Here's how the part is built. I have some questions about the finished solid (model axes, mm). A direction names the side the tool comes from. Round coordinates to 2 decimals unless told otherwise and drop trailing zeros. Write each loop counter-clockwise with the first axis right and the second up, starting at its lowest first coordinate (ties: lowest second). Pieces come first, ordered by that corner, then holes. Notation, with made-up numbers: (45.5, 40.25) -> (77.5, 40.25) arc R8 cw to (77.5, 45.25) -> close; hole circle Ø2 at (-11, 47). An arc over 180 degrees is marked (long way). Answer in a Markdown table with one row per item. Add a question column.
from build123d import *

# Parameters (mm, degrees)
SKETCH1_R           = 3.25
BOSS_EXTRUDE1_DEPTH = 10
SKETCH2_R           = 1.75
CUT_EXTRUDE1_DEPTH  = 2.5
SKETCH6_R           = 5
BOSS_EXTRUDE2_DEPTH = 5
BOSS_EXTRUDE3_DEPTH = 1


with BuildPart() as part:
    # Sketch1 → Boss-Extrude1 (new body)
    with BuildSketch(Plane(origin=(0, 0, 0), x_dir=(1, 0, 0), z_dir=(0, 1, 0))):
        Circle(SKETCH1_R)
    extrude(amount=BOSS_EXTRUDE1_DEPTH)

    # Sketch2 → Cut-Extrude1 (cut)
    with BuildSketch(Plane.XZ):
        Circle(SKETCH2_R)
    extrude(amount=-CUT_EXTRUDE1_DEPTH, mode=Mode.SUBTRACT)

    # Sketch6 → Boss-Extrude2 (add)
    with BuildSketch(Plane(origin=(0, 10, 0), x_dir=(1, 0, 0), z_dir=(0, 1, 0))):
        Circle(SKETCH6_R)
    extrude(amount=BOSS_EXTRUDE2_DEPTH)

    # Sketch9 → Boss-Extrude3 (add)
    with BuildSketch(Plane(origin=(0, 15, 0), x_dir=(1, 0, 0), z_dir=(0, 1, 0))):
        Polygon((-2.9, 2.9), (-2.9, -2.9), (2.9, 0), align=None)
    extrude(amount=BOSS_EXTRUDE3_DEPTH)


solid = part.part
Item 1: If we section it at C-C on y = 3.75: Please give me the cut outline in (x, z), then the cut area to 3 significant figures.
Item 2: On a 3-axis mill with a long thin cutter (end or side, diameter ignored), from which of +Z, -Z, +X, -X, +Y, -Y can I reach the whole of each face in a straight line? I mean faces 1 (the flat face through (1.4, 0, 1.4)), 2 (the flat face through (-2.9, 15.5, 0)), 3 (the flat face through (-1, 16, 0)), 4 (the flat face through (1, 10, 3.3)), 5 (the flat face through (0.04, 15.49, -1.43)). Say none if no direction works.
Item 3: If we section it at A-A on x = 0: Please give me the cut outline in (y, z).
Item 4: I need wall thicknesses on line 1 along Z through (x, y) = (0, 1.9); line 2 along Y through (x, z) = (-4.5, -0.75); line 3 along Y through (x, z) = (1, -1.25). Which ranges of each line are inside material? Lowest first, please. Write a range as from..to.
Item 5: If we section it at D-D on x = -2: Please give me the cut outline in (y, z).
Item 6: If we section it at B-B on z = -1.25: Please give me the cut outline in (x, y).
Item 7: If we mould it in two halves opening along Z, with no side actions, what happens to faces 6 (the cylindrical face through (1.617, 1.232, -0.67)), 7 (the cylindrical face through (-2.579, 4.93, 1.978)), 8 (the flat face through (0, 2.5, 0)), 9 (the flat face through (-0.04, 15.49, 1.47))? For each: pulls with the +Z half, pulls with the -Z half, needs draft (parallel to the pull), parting line crosses it, or undercut.
Item 8: For P1, Ø2, axis at x = 0, y = 6.5, coming from the +Z side; P2, Ø0.8, axis at y = 15.5, z = 0, coming from the -X side; P3, Ø6, axis at y = 6.5, z = 2.5, coming from the +X side, each with a flat end and sliding along its axis, tell me the tip position at first contact or that it passes through.
Results list:
| question | item | result |
|---|---|---|
| 1 | outline | circle Ø6.5 at (0, 0) |
| 1 | area | 33.2 mm² |
| 2 | face 1 | +Z, -Z, +X, -X, -Y |
| 2 | face 2 | +Z, -Z, -X, +Y |
| 2 | face 3 | +Z, -Z, +X, -X, +Y |
| 2 | face 4 | -Y |
| 2 | face 5 | -Z, +X, +Y |
| 3 | outline | (0, -3.25) -> (10, -3.25) -> (10, -5) -> (15, -5) -> (15, -1.45) -> (16, -1.45) -> (16, 1.45) -> (15, 1.45) -> (15, 5) -> (10, 5) -> (10, 3.25) -> (0, 3.25) -> (0, 1.75) -> (2.5, 1.75) -> (2.5, -1.75) -> (0, -1.75) -> close |
| 4 | line 1 | -3.25..-1.75, 1.75..3.25 |
| 4 | line 2 | 10..15 |
| 4 | line 3 | 2.5..15 |
| 5 | outline | (0, -2.56) -> (10, -2.56) -> (10, -4.58) -> (15, -4.58) -> (15, -2.45) -> (16, -2.45) -> (16, 2.45) -> (15, 2.45) -> (15, 4.58) -> (10, 4.58) -> (10, 2.56) -> (0, 2.56) -> close |
| 6 | outline | (-4.84, 10) -> (-3, 10) -> (-3, 0) -> (-1.22, 0) -> (-1.22, 2.5) -> (1.22, 2.5) -> (1.22, 0) -> (3, 0) -> (3, 10) -> (4.84, 10) -> (4.84, 15) -> (0.4, 15) -> (0.4, 16) -> (-2.9, 16) -> (-2.9, 15) -> (-4.84, 15) -> close |
| 7 | face 6 | undercut |
| 7 | face 7 | parting line crosses it |
| 7 | face 8 | undercut |
| 7 | face 9 | pulls with the +Z half |
| 8 | P1 | z = 3.25 |
| 8 | P2 | x = -2.9 |
| 8 | P3 | x = 3.25 |
